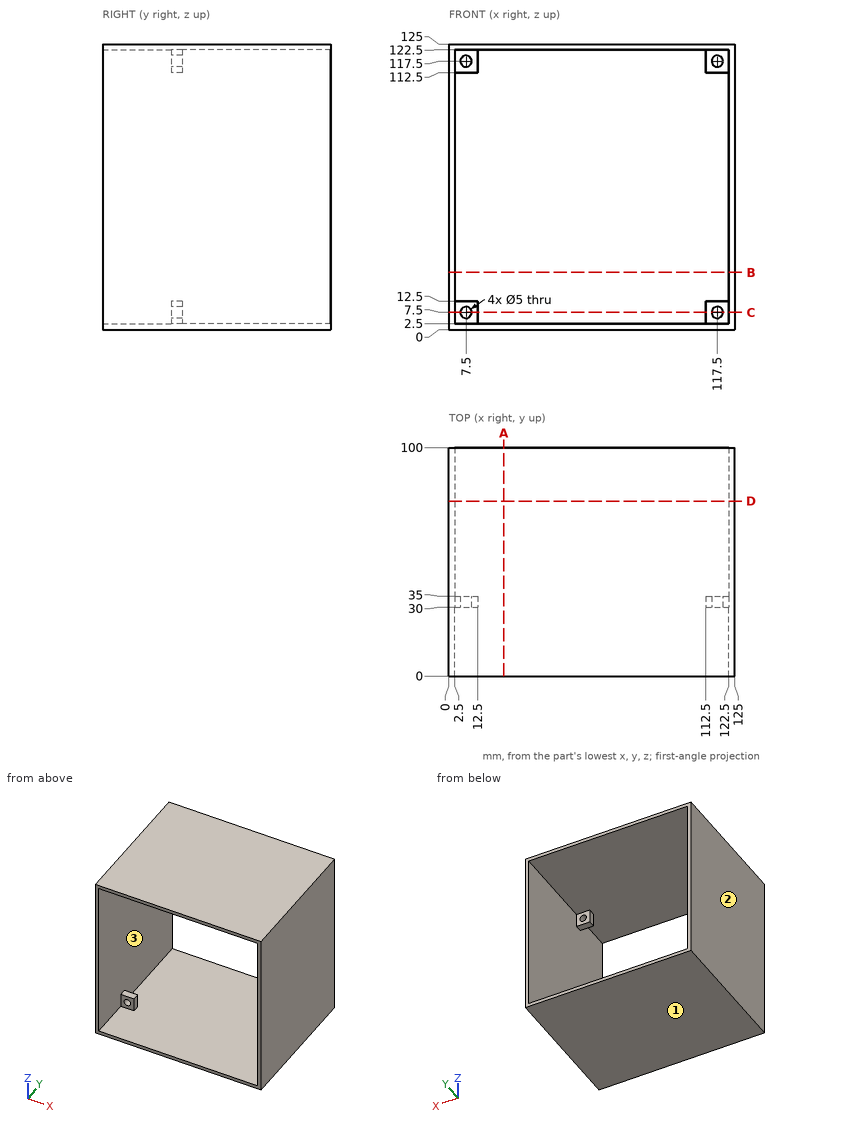
Can you work these out from the drawing? Everything is in mm from the part's minimum corner. Coordinates: 2 decimals unless noted, no trailing zeros. Loops run counter-clockwise (first coordinate to the right, second up) from the corner with the lowest first, then second, coordinate; pieces in that order, holes last.
1) Please list where these lines run through material, in increasing order: line 1 along X through (y, z) = (32.8, 117.5); line 2 along Z through (x, y) = (57.5, 53.5).
Reported:
line 1: x = 0 to 5, 10 to 12.5, 112.5 to 115, 120 to 125
line 2: z = 0 to 2.5, 122.5 to 125
2) Imagine slicing it at B-B (z = 25). List the corners of the cut face in (x, y) for me.
Reported:
outline: (0, 0) - (2.5, 0) - (2.5, 100) - (0, 100) - close; (122.5, 0) - (125, 0) - (125, 100) - (122.5, 100) - close
3) Will these pins go through, and if not, where does the flat tip stop? pin 1 Ø3 at (x, z) = (8.5, 9) entering from -Y; pin 2 Ø3 at (x, z) = (118, 5.5) entering from +Y.
Reported:
pin 1: stops at y = 30
pin 2: stops at y = 35
4) Thinking about a two-plate mould opening in Z: for the marked faces 1, 2 and 3, which applies, released by +Z, released by -Z, zero draft, split by the parting line, or undercut?
Reported:
face 1: released by -Z
face 2: zero draft
face 3: undercut
5) Imagine slicing it at D-D (y = 76.5). List the corners of the cut face in (x, z) for me.
Reported:
outline: (0, 0) - (125, 0) - (125, 125) - (0, 125) - close; hole (2.5, 2.5) - (122.5, 2.5) - (122.5, 122.5) - (2.5, 122.5) - close
6) Imagine slicing it at C-C (z = 7.5). List the corners of the cut face in (x, y) for me.
Reported:
outline: (0, 0) - (2.5, 0) - (2.5, 30) - (5, 30) - (5, 35) - (2.5, 35) - (2.5, 100) - (0, 100) - close; (10, 30) - (12.5, 30) - (12.5, 35) - (10, 35) - close; (112.5, 30) - (115, 30) - (115, 35) - (112.5, 35) - close; (120, 30) - (122.5, 30) - (122.5, 0) - (125, 0) - (125, 100) - (122.5, 100) - (122.5, 35) - (120, 35) - close
7) Imagine slicing it at A-A (x = 24). List the corners of the cut face in (y, z) for me.
Reported:
outline: (0, 0) - (100, 0) - (100, 2.5) - (0, 2.5) - close; (0, 122.5) - (100, 122.5) - (100, 125) - (0, 125) - close
